Geometry: see drawing. Coordinates: mm, zero at the bounding-box minimum. A direction names the side the tool comes from. Give positions to 0.01 mm unless a question says otherwise; leave off trailing zeros. Answer as a JSON object with one key per item and string values. Group by question number.
1. Set-up query: the marked faces 4, 5 and 6. Return all of +Z, -Z, +X, -X, +Y, -Y with unobstructed straight access to the full face (end or side cutting, diameter ignored); none if empty.
2. Pin query (flat end, axial travel): P1, Ø5, axis at y = 47.5, z = 27, coming from the +X side; P2, Ø8, axis at x = 10.5, y = 36.5, coming from the -Z side; P3, Ø8, axis at y = 41.5, z = 5.5, coming from the +X side; P4, Ø10, axis at x = 20.5, z = 20.5, coming from the +Y side. Return the tip coordinate at first contact, or that it passes through.
3. Pull-direction query (X, two-part tool) for the marked faces 1, 2 and 3; classes: +X half, -X half, draft (parallel to the pull), parting line (faces both ways), or undercut.
4. Material intervals for L1, parallel to Z at x = 4.25, y = 57.15 (1 decimal); L2, parallel to X at y = 31, z = 28, sorted ascending. Write a range as [from, to].
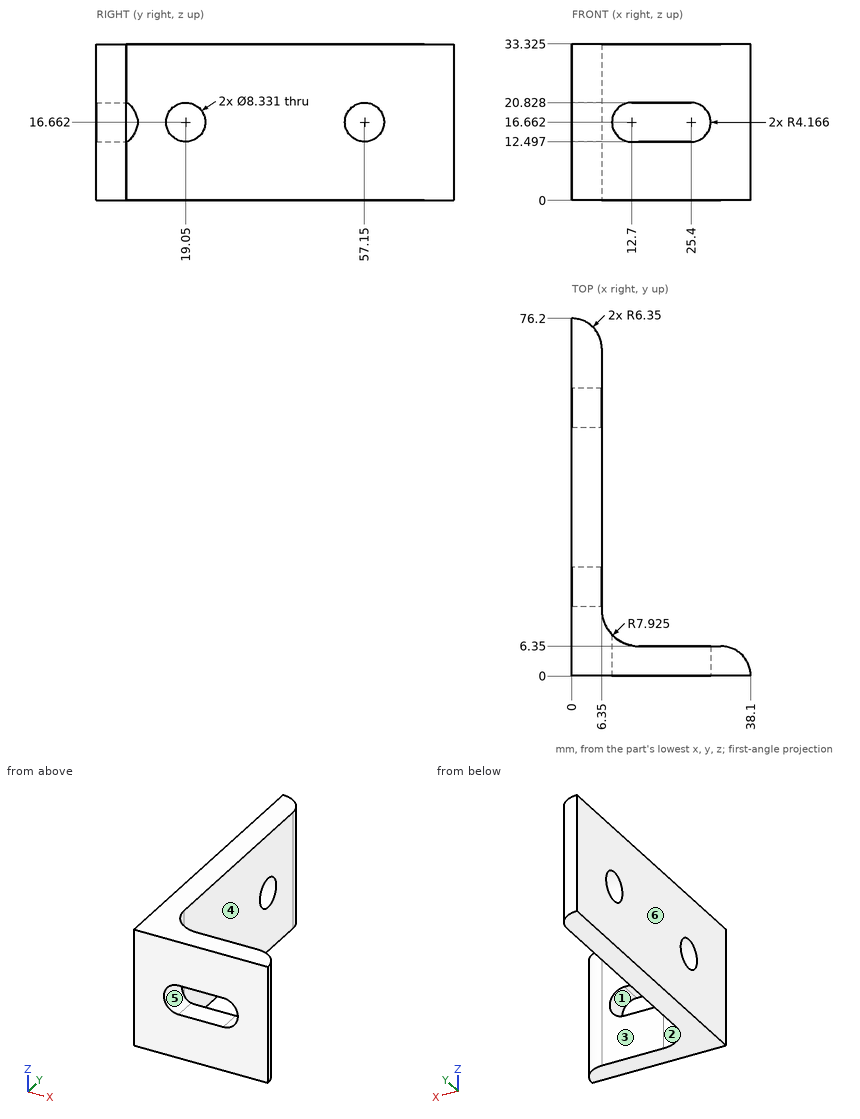
Answer sheet:
{
 "1": {"face 4": "+Z, -Z, +X, +Y", "face 5": "+Y, -Y", "face 6": "+Z, -Z, -X, +Y, -Y"},
 "2": {"P1": "x = 6.35", "P2": "through", "P3": "x = 6.35", "P4": "y = 6.35"},
 "3": {"face 1": "undercut", "face 2": "+X half", "face 3": "draft"},
 "4": {"L1": "[0, 12.5], [20.8, 33.3]", "L2": "[0, 6.35]"}
}
